from build123d import *

# Parameters (mm, degrees)
SKETCH3_W           = 12.8
SKETCH3_H           = 6.5
BOSS_EXTRUDE1_DEPTH = 5.8
SKETCH4_W           = 0.4
SKETCH4_H           = 0.375
SKETCH4_H_2         = 0.75
BOSS_EXTRUDE2_DEPTH = 3.5
FILLET1_R           = 0.2
CUT_EXTRUDE1_REACH  = 12.962
SKETCH5_R           = 0.7
BOSS_EXTRUDE4_START = -1.4
BOSS_EXTRUDE4_DEPTH = 3
FILLET2_R           = 0.5


with BuildPart() as part:
    # Sketch3 → Boss-Extrude1 (new body)
    with BuildSketch(Plane(origin=(0, 0, 0), x_dir=(0, 0, -1), z_dir=(1, 0, 0))):
        Rectangle(SKETCH3_W, SKETCH3_H)
    extrude(amount=BOSS_EXTRUDE1_DEPTH)

    # Sketch4 → Boss-Extrude2 (add)
    with BuildSketch(Plane.XZ.offset(3.25)):
        with Locations((2.9, -0.1875)):
            Rectangle(SKETCH4_W, SKETCH4_H)
        with Locations((2.9, 0.1875)):
            Rectangle(SKETCH4_W, SKETCH4_H)
        with Locations((2.9, 5.08)):
            Rectangle(SKETCH4_W, SKETCH4_H_2)
        with Locations((2.9, -5.08)):
            Rectangle(SKETCH4_W, SKETCH4_H_2)
    extrude(amount=BOSS_EXTRUDE2_DEPTH)

    # Fillet1
    fillet1_edges = [part.edges().sort_by_distance(p)[0] for p in [
        (3.1, -6.75, 0),
        (2.9, -6.75, 0.375),
        (2.7, -6.75, 0),
        (2.9, -6.75, -0.375),
        (3.1, -6.75, 5.08),
        (2.9, -6.75, 5.455),
        (2.7, -6.75, 5.08),
        (2.9, -6.75, 4.705),
        (2.9, -6.75, -4.705),
        (2.7, -6.75, -5.08),
        (2.9, -6.75, -5.455),
        (3.1, -6.75, -5.08),
    ]]
    fillet(fillet1_edges, radius=FILLET1_R - 0.0001)  # a hair under: the kernel refuses the full size

    # Sketch5 → Cut-Extrude1 (cut, up to next)
    with BuildSketch(Plane.ZY, mode=Mode.PRIVATE) as cut_extrude1_sk1:
        with Locations((-3.25, -1.75)):
            Circle(SKETCH5_R)
    cut_extrude1_tool1 = extrude(cut_extrude1_sk1.sketch, amount=-CUT_EXTRUDE1_REACH, mode=Mode.PRIVATE) & part.part
    # Sketch5 → Cut-Extrude1 (cut, up to next)
    with BuildSketch(Plane.ZY, mode=Mode.PRIVATE) as cut_extrude1_sk2:
        with Locations((3.25, -1.75)):
            Circle(SKETCH5_R)
    cut_extrude1_tool2 = extrude(cut_extrude1_sk2.sketch, amount=-CUT_EXTRUDE1_REACH, mode=Mode.PRIVATE) & part.part
    add(cut_extrude1_tool1.solids().sort_by_distance((0, -1.75, -3.25))[0], mode=Mode.SUBTRACT)
    add(cut_extrude1_tool2.solids().sort_by_distance((0, -1.75, 3.25))[0], mode=Mode.SUBTRACT)

    # Sketch6 → Boss-Extrude4 (add)
    with BuildSketch(Plane.ZY.offset(BOSS_EXTRUDE4_START)):
        Polygon((-5.455, 3.25), (7.55, 5.05), (7.577420264, 4.851888594), (-3.996224829, 3.25), align=None)
    extrude(amount=-BOSS_EXTRUDE4_DEPTH)

    # Fillet2
    fillet2_edges = [part.edges().sort_by_distance(p)[0] for p in [
        (5.8, 0, 6.4),
        (5.8, -3.25, 0),
        (5.8, 0, -6.4),
        (0, -3.25, 0),
        (0, 0, 6.4),
        (0, 3.25, 0),
        (0, 0, -6.4),
        (2.9, -3.25, -6.4),
        (2.9, -3.25, 6.4),
        (2.9, 3.25, 6.4),
        (2.9, 3.25, -6.4),
        (5.8, 3.25, 0),
    ]]
    fillet(fillet2_edges, radius=FILLET2_R)


solid = part.part
Can you work these out from the model? Positions are in its coordinate system, mm. Give positions to 0.01 mm unless a question says otherwise; leave off trailing zeros. Loops run counter-clockwise (first coordinate to the right, second up) from the corner with the lowest first, then second, coordinate; pieces in that order, holes last. Notation, with made-up numbers: (65, -22) - (73, -22) arc R16 ccw to (73, -12) - close; hole circle Ø6 at (10.25, -13). An arc over 180 degrees is marked (long way). Return JSON: item names as keys, results as strings.
1. I'm going to push flat-ended pins straight in: pin 1 Ø2 at (x, y) = (4, -2.5) entering from +Z; pin 2 Ø0.8 at (y, z) = (-5.5, -5) entering from -X; pin 3 Ø3 at (x, y) = (1.5, -5.5) entering from +Z (3 decimals). Where does each tip first touch, or does it pass through?
Output values:
{"pin 1": "stops at z = 6.4", "pin 2": "stops at x = 2.7", "pin 3": "stops at z = 5.455"}
2. I want a section at B-B on y = -1.75. Please give me the cut outline in (x, z).
Output values:
{"outline": "(0, -5.9) arc R0.5 ccw to (0.5, -6.4) - (5.3, -6.4) arc R0.5 ccw to (5.8, -5.9) - (5.8, -3.95) - (0, -3.95) - close; (0, -2.55) - (5.8, -2.55) - (5.8, 2.55) - (0, 2.55) - close; (0, 3.95) - (5.8, 3.95) - (5.8, 5.9) arc R0.5 ccw to (5.3, 6.4) - (0.5, 6.4) arc R0.5 ccw to (0, 5.9) - close"}
3. I want a section at C-C on z = 3.25. Please give me the cut outline in (x, y), and give its area (3 significant figures).
Output values:
{"outline": "(0, -2.75) arc R0.5 ccw to (0.5, -3.25) - (5.3, -3.25) arc R0.5 ccw to (5.8, -2.75) - (5.8, -2.45) - (0, -2.45) - close; (0, -1.05) - (5.8, -1.05) - (5.8, 2.75) arc R0.5 ccw to (5.3, 3.25) - (0.5, 3.25) arc R0.5 ccw to (0, 2.75) - close; (1.4, 4.25) - (4.4, 4.25) - (4.4, 4.45) - (1.4, 4.45) - close", "area": "30.0 mm²"}
4. I want a section at A-A on x = 4.6. Please give me the cut outline in (y, z).
Output values:
{"outline": "(-3.25, -5.9) arc R0.5 ccw to (-2.75, -6.4) - (2.75, -6.4) arc R0.5 ccw to (3.25, -5.9) - (3.25, 5.9) arc R0.5 ccw to (2.75, 6.4) - (-2.75, 6.4) arc R0.5 ccw to (-3.25, 5.9) - close; hole circle Ø1.4 at (-1.75, -3.25); hole circle Ø1.4 at (-1.75, 3.25)"}
5. We'd pull the mould along Y, two halves only. Please class faces 1 (the face through (2.88, 4.06, 1.87)), 2 (the face through (3, 0, 6.4)), 3 (the face through (2.879, 4.137, 0.956)): +Y half, -Y half, draft (parallel to the pull), parting line (faces both ways), or undercut.
Output values:
{"face 1": "undercut", "face 2": "draft", "face 3": "+Y half"}
6. If I drill on line 1 (Y direction, x = 2.5, z = 3.25); line 2 (Z direction, x = 3.3, y = -0.5); line 3 (Z direction, x = 1.85, y = -1.5), over which ranges is the centre line in solid material (lowest first)?
Output values:
{"line 1": "y = -3.25 to -2.45, -1.05 to 3.25, 4.25 to 4.45", "line 2": "z = -6.4 to 6.4", "line 3": "z = -6.4 to -3.9, -2.6 to 2.6, 3.9 to 6.4"}
7. I want a section at D-D on y = 0.25. Please give me the cut outline in (x, z), and give its area (3 significant figures).
Output values:
{"outline": "(0, -5.9) arc R0.5 ccw to (0.5, -6.4) - (5.3, -6.4) arc R0.5 ccw to (5.8, -5.9) - (5.8, 5.9) arc R0.5 ccw to (5.3, 6.4) - (0.5, 6.4) arc R0.5 ccw to (0, 5.9) - close", "area": "74.0 mm²"}
